Design review of the part built by this model. Coordinates are the model's own, in mm. A direction names the side the tool comes from. Coordinates: 2 decimals unless noted, no trailing zeros. Write each loop counter-clockwise with the first axis right and the second up, starting at its lowest first coordinate (ties: lowest second). Pieces come first, ordered by that corner, then holes. Notation, with made-up numbers: M 55.5,-13 L 106.5,-13 A30 cw 106.5,25 Z; hole C 57.25,21 d4. An arc over 180 degrees is marked long. Write item = value, one per line.
```python
from build123d import *

# Parameters (mm, degrees)
SKETCH1_R           = 2
BOSS_EXTRUDE1_DEPTH = 6
CUT_EXTRUDE1_DEPTH  = 2.3
SKETCH3_R           = 3.1
BOSS_EXTRUDE2_DEPTH = 5
BOSS_EXTRUDE3_DEPTH = 5
FILLET1_R           = 7.5
BOSS_EXTRUDE4_DEPTH = 5
CUT_EXTRUDE2_REACH  = 139.089


with BuildPart() as part:
    # Sketch1 → Boss-Extrude1 (new body)
    with BuildSketch(Plane(origin=(0, 0, 0), x_dir=(1, 0, 0), z_dir=(0, 1, 0))):
        with BuildLine():
            Line((26.846717088, 0), (37.5, 10.653282912))
            Line((37.5, 10.653282912), (37.5, 64.346717088))
            Line((37.5, 64.346717088), (26.846717088, 75))
            Line((26.846717088, 75), (32.928932188, 81.0822151))
            ThreePointArc((32.928932188, 81.0822151), (43.826834324, 83.249942613), (50, 74.011147288))
            Line((50, 74.011147288), (50, -12.5))
            Line((50, -12.5), (-50, -12.5))
            Line((-50, -12.5), (-50, 74.011147288))
            ThreePointArc((-50, 74.011147288), (-43.826834324, 83.249942613), (-32.928932188, 81.0822151))
            Line((-32.928932188, 81.0822151), (-26.846717088, 75))
            Line((-26.846717088, 75), (-37.5, 64.346717088))
            Line((-37.5, 64.346717088), (-37.5, 10.653282912))
            Line((-37.5, 10.653282912), (-26.846717088, 0))
            Line((-26.846717088, 0), (26.846717088, 0))
        make_face()
        with Locations(Location((35.70889245, 1.79110755, 0), (0, 0, 270))):
            Circle(SKETCH1_R, mode=Mode.SUBTRACT)
        with Locations(Location((-35.70889245, 1.79110755, 0), (0, 0, 90))):
            Circle(SKETCH1_R, mode=Mode.SUBTRACT)
        with Locations(Location((35.70889245, 73.20889245, 0), (0, 0, 270))):
            Circle(SKETCH1_R, mode=Mode.SUBTRACT)
        with Locations(Location((-35.70889245, 73.20889245, 0), (0, 0, 90))):
            Circle(SKETCH1_R, mode=Mode.SUBTRACT)
    extrude(amount=BOSS_EXTRUDE1_DEPTH)

    # Sketch2 → Cut-Extrude1 (cut)
    with BuildSketch(Plane.XZ):
        Polygon((-37.325473204, -70.40889245), (-38.942053957, -73.20889245), (-37.325473204, -76.00889245), (-34.092311696, -76.00889245), (-32.475730942, -73.20889245), (-34.092311696, -70.40889245), align=None)
        Polygon((-38.942053957, -1.79110755), (-37.325473204, -4.59110755), (-34.092311696, -4.59110755), (-32.475730942, -1.79110755), (-34.092311696, 1.00889245), (-37.325473204, 1.00889245), align=None)
        Polygon((34.092311696, 1.00889245), (32.475730942, -1.79110755), (34.092311696, -4.59110755), (37.325473204, -4.59110755), (38.942053957, -1.79110755), (37.325473204, 1.00889245), align=None)
        Polygon((32.475730942, -73.20889245), (34.092311696, -76.00889245), (37.325473204, -76.00889245), (38.942053957, -73.20889245), (37.325473204, -70.40889245), (34.092311696, -70.40889245), align=None)
    extrude(amount=-CUT_EXTRUDE1_DEPTH, mode=Mode.SUBTRACT)

    # Sketch3 → Boss-Extrude2 (add)
    with BuildSketch(Plane.XY.offset(12.5)):
        with BuildLine():
            Line((-50, 0), (50, 0))
            Line((50, 0), (50, -10))
            ThreePointArc((50, -10), (42.582009977, -47.796447301), (21.428571429, -79.985421222))
            ThreePointArc((21.428571429, -79.985421222), (0, -88.989794856), (-21.428571429, -79.985421222))
            ThreePointArc((-21.428571429, -79.985421222), (-42.582009977, -47.796447301), (-50, -10))
            Line((-50, -10), (-50, 0))
        make_face()
        with Locations((10, -10)):
            Circle(SKETCH3_R, mode=Mode.SUBTRACT)
        with Locations((-10, -10)):
            Circle(SKETCH3_R, mode=Mode.SUBTRACT)
    extrude(amount=-BOSS_EXTRUDE2_DEPTH)

    # Sketch4 → Boss-Extrude3 (add)
    with BuildSketch(Plane(origin=(0, 0, 7.5), x_dir=(-1, 0, 0), z_dir=(0, 0, -1))):
        with BuildLine():
            Line((-20.888972746, -10), (-20.888972746, 0))
            Line((-20.888972746, 0), (0, 0))
            Line((0, 0), (20.888972746, 0))
            Line((20.888972746, 0), (20.888972746, -10))
            ThreePointArc((20.888972746, -10), (15.559129957, -19.36300174), (4.787214825, -19.560156807))
            ThreePointArc((4.787214825, -19.560156807), (0, -18.339825037), (-4.787214825, -19.560156807))
            ThreePointArc((-4.787214825, -19.560156807), (-15.559129957, -19.36300174), (-20.888972746, -10))
        make_face()
        Polygon((-10, -4.111027254), (-15.1, -7.055513627), (-15.1, -12.944486373), (-10, -15.888972746), (-4.9, -12.944486373), (-4.9, -7.055513627), align=None, mode=Mode.SUBTRACT)
        Polygon((4.9, -7.055513627), (10, -4.111027254), (15.1, -7.055513627), (15.1, -12.944486373), (10, -15.888972746), (4.9, -12.944486373), align=None, mode=Mode.SUBTRACT)
    extrude(amount=BOSS_EXTRUDE3_DEPTH)

    # Fillet1
    fillet1_edges = [part.edges().sort_by_distance(p)[0] for p in [
        (-20.888972746, 0, 5),
        (20.888972746, 0, 5),
    ]]
    fillet(fillet1_edges, radius=FILLET1_R)

    # Sketch5 → Boss-Extrude4 (add)
    with BuildSketch(Plane(origin=(50, 0, 0), x_dir=(0, 0, -1), z_dir=(1, 0, 0))):
        Polygon((17.5, 0), (-7.5, 0), (-7.5, -25), align=None)
    boss_extrude4 = extrude(amount=-BOSS_EXTRUDE4_DEPTH)

    # Mirror1: Boss-Extrude4 across plane
    add(boss_extrude4.mirror(Plane(origin=(0, 0, 0), x_dir=(0, 0, 1), z_dir=(1, 0, 0))))

    # Sketch6 → Cut-Extrude2 (cut, up to next)
    with BuildSketch(Plane.XY.offset(7.5), mode=Mode.PRIVATE) as cut_extrude2_sk1:
        with BuildLine():
            Line((50, -25), (50, -10))
            ThreePointArc((50, -10), (49.71674876, -17.521304187), (48.868599666, -25))
            Line((48.868599666, -25), (50, -25))
        make_face()
    cut_extrude2_tool1 = extrude(cut_extrude2_sk1.sketch, amount=-CUT_EXTRUDE2_REACH, mode=Mode.PRIVATE) & part.part
    # Sketch6 → Cut-Extrude2 (cut, up to next)
    with BuildSketch(Plane.XY.offset(7.5), mode=Mode.PRIVATE) as cut_extrude2_sk2:
        with BuildLine():
            Line((-50, -10), (-50, -25))
            Line((-50, -25), (-48.868599666, -25))
            ThreePointArc((-48.868599666, -25), (-49.71674876, -17.521304187), (-50, -10))
        make_face()
    cut_extrude2_tool2 = extrude(cut_extrude2_sk2.sketch, amount=-CUT_EXTRUDE2_REACH, mode=Mode.PRIVATE) & part.part
    add(cut_extrude2_tool1.solids().sort_by_distance((49.660912, -21.254256, 7.5))[0], mode=Mode.SUBTRACT)
    add(cut_extrude2_tool2.solids().sort_by_distance((-49.660912, -21.254256, 7.5))[0], mode=Mode.SUBTRACT)


solid = part.part
```
Q1. The part is to be moulded in two halves that separate along X. For faces 6 (the flat face through (47.5, -12.7, -4.8)), 7 (the flat face through (32.099, 2.958, -5.252)), 8 (the flat face through (-50, 2, -21)), say which applies: +X half, -X half, draft (parallel to the pull), parting line (faces both ways), or undercut.
Check result:
face_6 = draft
face_7 = undercut
face_8 = -X half
Q2. For P1, Ø4, axis at x = -6.5, y = -33, coming from the -Z side; P2, Ø1.7, axis at x = 34.5, z = -1, coming from the -Y side; P3, Ø6, axis at x = -36.5, z = -72, coming from the -Y side, all flat-tipped, find the tip position at first contact; note any pin that passes through.
Check result:
P1 = 7.5
P2 = 2.3
P3 = 0
Q3. Consider section A-A, the plane z = -44.5. State the section outline as (x, y) points, and give its area (3 significant figures).
Check result:
outline = M -50,0 L -37.5,0 L -37.5,6 L -50,6 Z; M 37.5,0 L 50,0 L 50,6 L 37.5,6 Z
area = 150 mm²
Q4. Consider section C-C, the plane y = -39. State the section outline as (x, z) points.
Check result:
outline = M -45.7,7.5 L 45.7,7.5 L 45.7,12.5 L -45.7,12.5 Z
Q5. Wall thickness on line 1 (Z direction, x = -15, y = 1); line 2 (Z direction, x = 11.5, y = -54); line 3 (Y direction, x = 10, z = 9.65): over which ranges is each line inside the solid? List them lowest first.
Check result:
line_1 = 0 to 12.5
line_2 = 7.5 to 12.5
line_3 = -87.27 to -13.1, -6.9 to 6
Q6. Consider section B-B, the plane y = -11.5. State the section outline as (x, z) points.
Check result:
outline = M -49.99,-6 L -45,-6 L -45,7.5 L -20.79,7.5 L -20.79,2.5 L -15.1,2.5 L -15.1,7.5 L -12.71,7.5 L -12.71,12.5 L -49.99,12.5 Z; M -7.29,7.5 L -4.9,7.5 L -4.9,2.5 L 4.9,2.5 L 4.9,7.5 L 7.29,7.5 L 7.29,12.5 L -7.29,12.5 Z; M 12.71,7.5 L 15.1,7.5 L 15.1,2.5 L 20.79,2.5 L 20.79,7.5 L 45,7.5 L 45,-6 L 49.99,-6 L 49.99,12.5 L 12.71,12.5 Z
Q7. Machinability: for faces 1 (the flat face through (38, 2.3, -2)), 2 (the flat face through (7.414, -5.604, 5.035)), 3 (the flat face through (0, -10, 2.5)), 4 (the flat face through (-29.93, 2.958, -78.084)), 5 (the flat face through (-32.099, 2.958, -69.748)), which of the approach directions +Z, -Z, +X, -X, +Y, -Y give a long, thin tool a straight path to every point of the face, cutting with its end or side? Answer none if there is none.
Check result:
face_1 = -Y
face_2 = -Z
face_3 = -Z, -Y
face_4 = -Z, +Y, -Y
face_5 = +Y, -Y
